Source: CAD feature listing. Evaluate the final solid. Frame: model axes, mm. A direction names the side the tool comes from. Coordinates: 2 decimals unless noted, no trailing zeros. Loops run counter-clockwise (first coordinate to the right, second up) from the corner with the lowest first, then second, coordinate; pieces in that order, holes last. Notation, with made-up numbers: M 30.5,88.25 L 58.5,88.25 A27 ccw 58.5,109.25 Z; hole C 55.5,-24.75 d1. An arc over 180 degrees is marked long. One line per question, with ' | ' between items. Start each with the question number.
1. Pin query (flat end, axial travel): P1, Ø4, axis at x = -5.5, y = -9, coming from the +Z side; P2, Ø4, axis at x = -1.5, y = -14, coming from the -Z side; P3, Ø4, axis at x = -3, z = 20.5, coming from the -Y side. Return the tip coordinate at first contact, or that it passes through.
2. Access query for faces 5 (the flat face through (-3, -20.05, 0)), 6 (the flat face through (-3, -11, 17.5)), 7 (the cylindrical face through (-1.435, -15.046, -0.331)), 8 (the flat face through (-1, -3, -20)), 9 (the flat face through (-3, 0, 19)). Directions: +Z, -Z, +X, -X, +Y, -Y. A direction counts if a zero-diameter tool reaches every point of the face in a straight line with its end or side. Return the directions, or none.
3. Section query B-B, the plane z = 21.25. Output: boundary loops of the cut face in (x, y).
4. Mould query, pull axis X, two halves, no side actions, for faces 1 (the flat face through (0, -14, -1)), 2 (the cylindrical face through (-2.6, -1.5, 25)), 3 (the cylindrical face through (-2.319, -1.479, 22.886)), 4 (the cylindrical face through (1.216, -13.497, -0.297)). Classes: pulls with the +X half, pulls with the -X half, needs draft (parallel to the pull), parting line crosses it, or undercut.
5. Section query C-C, the plane y = -13. Output: boundary loops of the cut face in (x, z), and give its area (3 significant figures).
6. Section query A-A, the plane y = -2.5. Output: boundary loops of the cut face in (x, z).
7. Ray query, probe 1 along Z at (x, y) = (-4.25, -18); probe 2 along Z at (x, y) = (-2, -6.5); probe 3 along Z at (x, y) = (-0.25, -4.5). Return the intervals inside material, ascending.
8. Section query D-D, the plane z = 0. Output: boundary loops of the cut face in (x, y), and give its area (3 significant figures).
```python
from build123d import *

# Parameters (mm, degrees)
SKETCH1_W           = 10
SKETCH1_H           = 20.05
BOSS_EXTRUDE4_DEPTH = 17.5
SKETCH11_R          = 13.5
CUT_EXTRUDE5_DEPTH  = 29.42978192
SKETCH13_R          = 1.65
BOSS_EXTRUDE7_DEPTH = 3


with BuildPart() as part:
    # Sketch1 → Boss-Extrude4 (new, symmetric)
    with BuildSketch(Plane.XY):
        with Locations((-2.533836661, -10.025)):
            Rectangle(SKETCH1_W, SKETCH1_H)
    extrude(amount=BOSS_EXTRUDE4_DEPTH, both=True)

    # Sketch1_5 → Cut-Revolve4 (revolve, cut)
    with BuildSketch(Plane.XY):
        with BuildLine():
            Line((0, 15.05), (-2.83, 15.05))
            ThreePointArc((-2.83, 15.05), (-4.505197002, 7.607721109), (-5.067673322, 0))
            Line((-5.067673322, 0), (0, 0))
            Line((0, 0), (0, 15.05))
        make_face()
    revolve(axis=Axis((0, 0, 0), (-1, 0, 0)), mode=Mode.SUBTRACT)

    # Sketch11 → Cut-Extrude5 (cut, through all)
    with BuildSketch(Plane.ZY.offset(7.533836661)):
        Circle(SKETCH11_R)
    extrude(amount=-CUT_EXTRUDE5_DEPTH, mode=Mode.SUBTRACT)

    # Sketch13 → Boss-Extrude7 (add)
    # profile 1 of 2: a face of its own
    with BuildSketch(Plane(origin=(0, 0, 0), x_dir=(1, 0, 0), z_dir=(0, 1, 0))):
        with BuildLine():
            Line((2.466163339, 17.5), (-7.533836661, 17.5))
            Line((-7.533836661, 17.5), (-7.533836661, 20))
            ThreePointArc((-7.533836661, 20), (-2.533836661, 25), (2.466163339, 20))
            Line((2.466163339, 20), (2.466163339, 17.5))
        make_face()
        with Locations(Location((-2.533836661, 21.25, 0), (0, 0, 180))):
            Circle(SKETCH13_R, mode=Mode.SUBTRACT)
    # profile 2 of 2: a face of its own
    with BuildSketch(Plane(origin=(0, 0, 0), x_dir=(1, 0, 0), z_dir=(0, 1, 0))):
        with BuildLine():
            Line((2.466163339, -17.5), (-7.533836661, -17.5))
            Line((-7.533836661, -17.5), (-7.533836661, -20))
            ThreePointArc((-7.533836661, -20), (-2.533836661, -25), (2.466163339, -20))
            Line((2.466163339, -20), (2.466163339, -17.5))
        make_face()
        with Locations(Location((-2.533836661, -21.25, 0), (0, 0, 180))):
            Circle(SKETCH13_R, mode=Mode.SUBTRACT)
    extrude(amount=-BOSS_EXTRUDE7_DEPTH)


solid = part.part
```
Taken from the geometry:
1) P1: z = 17.5 | P2: z = -17.5 | P3: y = -3
2) face 5: +Z, -Z, +X, -X, -Y | face 6: +Z, +X, -X, -Y | face 7: +Y | face 8: -Z, +X, -X, -Y | face 9: +Z, -Z, +X, -X, +Y
3) outline: M -7.38,-3 L -4.18,-3 L -4.18,0 L -7.38,0 Z; M -0.88,-3 L 2.31,-3 L 2.31,0 L -0.88,0 Z
4) face 1: undercut | face 2: parting line crosses it | face 3: undercut | face 4: needs draft
5) outline: M -7.53,-17.5 L 2.47,-17.5 L 2.47,-3.64 L 0,-3.64 L 0,-7.58 L -2.83,-7.58 A50.07 cw -3.28,-3.64 L -7.53,-3.64 Z; M -7.53,3.64 L -3.28,3.64 A50.07 cw -2.83,7.58 L 0,7.58 L 0,3.64 L 2.47,3.64 L 2.47,17.5 L -7.53,17.5 Z | area: 253 mm^2
6) outline: M -7.53,-20 A5 ccw 2.47,-20 L 2.47,-13.27 L 0,-13.27 L 0,-14.84 L -2.83,-14.84 A51.67 cw -3.28,-13.27 L -7.53,-13.27 Z; M -7.53,13.27 L -3.28,13.27 A51.67 cw -2.83,14.84 L 0,14.84 L 0,13.27 L 2.47,13.27 L 2.47,20 A5 ccw -7.53,20 Z; hole C -2.53,-21.25 d3.3; hole C -2.53,21.25 d3.3
7) probe 1: -17.5 to 17.5 | probe 2: -17.5 to -13.57, 13.57 to 17.5 | probe 3: -17.5 to -14.36, 14.36 to 17.5
8) outline: M -7.53,-20.05 L 2.47,-20.05 L 2.47,-13.5 L 0,-13.5 L 0,-15.05 L -2.83,-15.05 A51.73 cw -3.28,-13.5 L -7.53,-13.5 Z | area: 60.8 mm^2
